Geometry check sheet. Reference: drawing and pictorial views, mm from the part's lowest x, y, z. A direction names the side the tool comes from. Round coordinates to 2 decimals unless told otherwise and drop trailing zeros. Loops run counter-clockwise (first coordinate to the right, second up) from the corner with the lowest first, then second, coordinate; pieces in that order, holes last. Notation, with made-up numbers: (-17.5, 37.5) -> (-5.5, 37.5) arc R29 ccw to (-5.5, 67.5) -> close; hole circle Ø2 at (73, 19). An arc over 180 degrees is marked (long way). Use one line per item in the form item = value. Start each with the question number.
(1) Go/stop test with flat-tipped pins: pin 1 (3 mm diameter, centred on y = 4, z = 17, fed in from -X); pin 2 (6 mm diameter, centred on x = 73, y = 8.5, fed in from -Z); pin 3 (5.5 mm diameter, centred on x = 40.5, z = 17.5, fed in from +Y). Record where each tip stops, or that it passes through.
(2) Set-up check for the marked faces 5, 6 and 7: record each of +Z, -Z, +X, -X, +Y, -Y from which the full face is reachable in a straight line by a thin tool's end or side.
(3) Material ranges on probe 1 along Y at (x, z) = (69, 41.4); probe 2 along X at (y, z) = (8.25, 41.5); probe 3 along Z at (x, y) = (67.5, 1.5), recorded low to high. Write a range as [from, to].
(4) Sectioned sample at C-C (z = 41). Record the cut outline in (x, y).
(5) Sectioned sample at D-D (y = 6). Record the cut outline in (x, z) (3 decimals).
(6) Sectioned sample at A-A (x = 69). Record the cut outline in (y, z).
(7) Sectioned sample at B-B (y = 10). Record the cut outline in (x, z) (3 decimals), and give its area (4 significant figures).
(8) Draft check along Z on the marked faces 1, 2, 3 and 4. Enter one of: released by +Z, released by -Z, zero draft, split by the parting line, or undercut.
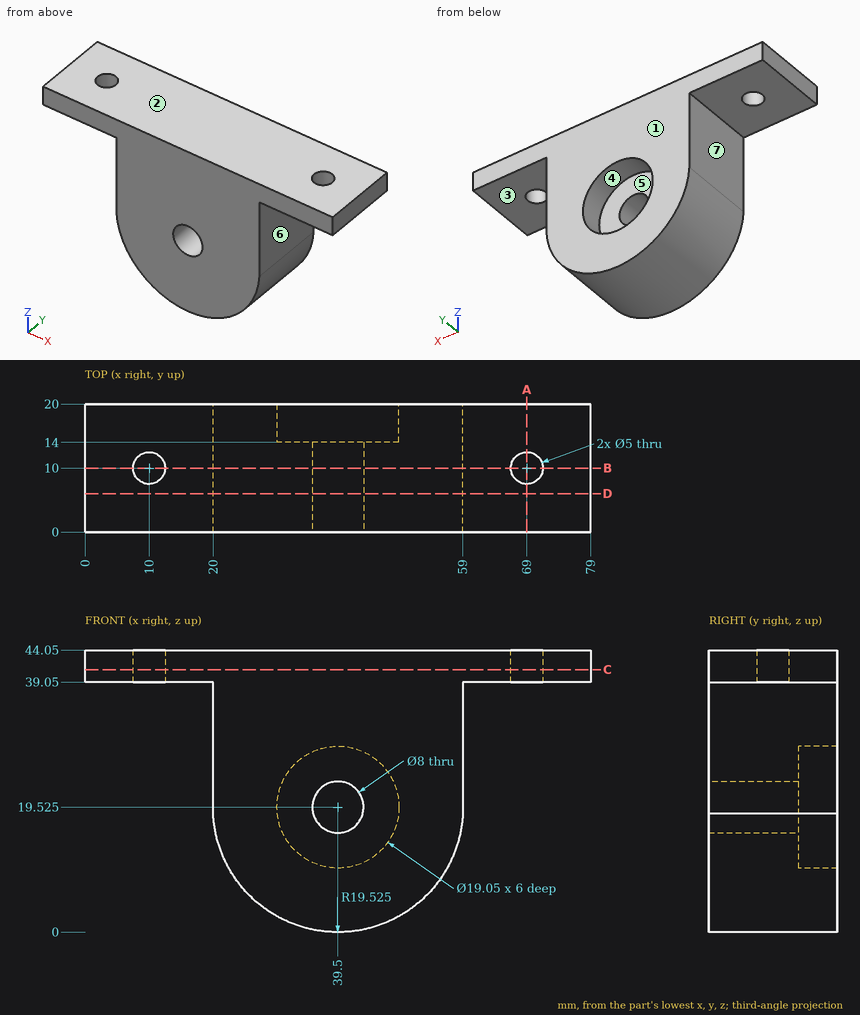
Checks:
q1.pin_1 = 20
q1.pin_2 = 39.05
q1.pin_3 = 14
q2.face_5 = +Y
q2.face_6 = -Z, +X, +Y, -Y
q2.face_7 = -Z, -X, +Y, -Y
q3.probe_1 = [0, 7.5], [12.5, 20]
q3.probe_2 = [0, 8.21], [11.79, 67.21], [70.79, 79]
q3.probe_3 = [39.05, 44.05]
q4.outline = (0, 0) -> (79, 0) -> (79, 20) -> (0, 20) -> close; hole circle Ø5 at (10, 10); hole circle Ø5 at (69, 10)
q5.outline = (0, 39.05) -> (20, 39.05) -> (20, 18.537) arc R19.525 ccw to (59, 18.537) -> (59, 39.05) -> (79, 39.05) -> (79, 44.05) -> (0, 44.05) -> close; hole circle Ø8 at (39.5, 19.525)
q6.outline = (0, 39.05) -> (7.5, 39.05) -> (7.5, 44.05) -> (0, 44.05) -> close; (12.5, 39.05) -> (20, 39.05) -> (20, 44.05) -> (12.5, 44.05) -> close
q7.outline = (0, 39.05) -> (7.5, 39.05) -> (7.5, 44.05) -> (0, 44.05) -> close; (12.5, 39.05) -> (20, 39.05) -> (20, 18.537) arc R19.525 ccw to (59, 18.537) -> (59, 39.05) -> (66.5, 39.05) -> (66.5, 44.05) -> (12.5, 44.05) -> close; (71.5, 39.05) -> (79, 39.05) -> (79, 44.05) -> (71.5, 44.05) -> close; hole circle Ø8 at (39.5, 19.525)
q7.area = 1,655 mm2
q8.face_1 = zero draft
q8.face_2 = released by +Z
q8.face_3 = released by -Z
q8.face_4 = undercut
